Can you work these out from the model? Positions are in its coordinate system, mm. Coordinates: 2 decimals unless noted, no trailing zeros. Answer in a Markdown table with one row per item. Add a question column.
1. We'd pull the mould along X, two halves only. Please class faces 1 (the face through (0, -101.6, 35)), 2 (the face through (21.431, -36, 33)), 3 (the face through (0, -152.4, 47)), 4 (the face through (-1.24, -127.36, 44.37)): pulls with the +X half, pulls with the -X half, needs draft (parallel to the pull), parting line crosses it, or undercut.
2. Will these pins go through, and if not, where does the flat tip stop? pin 1 (9.5 mm diameter, centred on x = -3.5, z = 32.5, fed in from -Y); pin 2 (12 mm diameter, centred on x = -13.5, y = -12.5, fed in from +Z); pin 3 (2 mm diameter, centred on x = -5.5, z = 54.5, fed in from +Y).
3. If I drill on line 1 along Z through (x, y) = (0, -127); line 2 along Z through (x, y) = (0, -121.5); line 3 along Z through (x, y) = (-13.5, -98.5), over which ranges is the centre line in solid material (lowest first)? Write a range as [from, to].
from build123d import *

# Parameters (mm, degrees)
F1_DEPTH = 21.43125
F2_R     = 9.525
F3_DEPTH = 50.8
F8_DEPTH = 56.3


# Not quite as in the source:
# - ends of sketch curves that miss each other by under 0.0002 mm in the source are joined


with BuildPart() as f1:
    # F0 (on Right) → F1 (new body, symmetric)
    with BuildSketch(Plane.YZ):
        Polygon((-152.4, 69.85), (-152.4, 0), (152.4, 0), (152.4, 19.05), align=None)
    extrude(amount=F1_DEPTH, both=True)

    # F2 (on face) → F3 (cut)
    with BuildSketch(Plane.XZ.offset(152.4)):
        with Locations((0, 34.925)):
            Circle(F2_R)
    extrude(amount=-F3_DEPTH, mode=Mode.SUBTRACT)

    # F5 (on face) → F8 (cut)
    with BuildSketch(Plane.YZ.offset(21.43125)):
        with BuildLine():
            add(Edge.make_bspline(
                [(-94.6281477809, 51.2691959739), (-96.0952206694, 52.0179937663), (-97.562293558, 52.7667915588), (-99.0539994454, 53.491879309)],
                knots=[0, 0, 0, 0, 0.1035282224, 0.1035282224, 0.1035282224, 0.1035282224], degree=3))
            add(Edge.make_bspline(
                [(-94.6281477809, 51.2691959739), (-88.9739529123, 49.8775010567), (-83.3197580522, 48.4858061416), (-73.0600804397, 46.9911508307)],
                knots=[0, 0, 0, 0, 0.1804237123, 0.1804237123, 0.1804237123, 0.1804237123], degree=3))
            add(Edge.make_bspline(
                [(11.0397725003, 37.6377859426), (-20.7191231776, 41.240284312), (-53.8117553476, 44.4768553148), (-73.0600804397, 46.9911508307)],
                knots=[0.3821429542, 0.3821429542, 0.3821429542, 0.3821429542, 0.5639196837, 0.5639196837, 0.5639196837, 0.5639196837], degree=3))
            add(Edge.make_bspline(
                [(11.0397725003, 37.6377859426), (19.8326583687, 36.6506728683), (28.6537852654, 35.611343032), (37.2394360057, 34.5120057533)],
                knots=[0.5008053198, 0.5008053198, 0.5008053198, 0.5008053198, 0.5858071806, 0.5858071806, 0.5858071806, 0.5858071806], degree=3))
            add(Edge.make_bspline(
                [(151.5644788742, 15.5920218676), (140.3358248303, 17.736038831), (112.6697575345, 23.0186414795), (69.4706003693, 30.4232191611), (37.2394360057, 34.5120057533)],
                knots=[0, 0, 0, 0, 0.1343010577, 0.3309018237, 0.3309018237, 0.3309018237, 0.3309018237], degree=3))
            Line((151.5644788742, 15.5920218676), (-152.4, 15.5920218676))
            Line((-152.4, 15.5920218676), (-152.4, 0))
            Line((-152.4, 0), (152.4, 0))
            Line((152.4, 0), (152.4, 19.05))
            Line((152.4, 19.05), (-152.4, 69.85))
            Line((-152.4, 69.85), (-152.4, 58.510940522))
            add(Edge.make_bspline(
                [(-152.1597802639, 58.510940522), (-152.2398342689, 58.510940522), (-152.3198882739, 58.510940522), (-152.4, 58.510940522)],
                knots=[0, 0, 0, 0, 0.240162015, 0.240162015, 0.240162015, 0.240162015], degree=3))
            add(Edge.make_bspline(
                [(-126.880271242, 59.893312547), (-131.0252775202, 59.9641176604), (-141.283309107, 59.6280745769), (-148.0759439731, 58.9303957414), (-152.1597802639, 58.510940522)],
                knots=[0.8645812396, 0.8645812396, 0.8645812396, 0.8645812396, 0.9185841637, 1, 1, 1, 1], degree=3))
            add(Edge.make_bspline(
                [(-114.7441045161, 58.9132569857), (-118.4444301689, 59.5720764958), (-122.5362126789, 59.8541063708), (-126.880271242, 59.893312547)],
                knots=[0.431288265, 0.431288265, 0.431288265, 0.431288265, 0.6334912794, 0.6334912794, 0.6334912794, 0.6334912794], degree=3))
            add(Edge.make_bspline(
                [(-99.0539994454, 53.491879309), (-99.5844007901, 53.7839672826), (-103.1690308471, 55.7243154808), (-108.8461739052, 57.9235356565), (-114.7441045161, 58.9132569857)],
                knots=[0.7100922868, 0.7100922868, 0.7100922868, 0.7100922868, 0.7255634136, 0.8104095628, 0.8104095628, 0.8104095628, 0.8104095628], degree=3))
        make_face()
    extrude(amount=-F8_DEPTH, mode=Mode.SUBTRACT)


solid = f1.part
Answers follow:
| question | item | result |
|---|---|---|
| 1 | face 1 | undercut |
| 1 | face 2 | pulls with the +X half |
| 1 | face 3 | needs draft |
| 1 | face 4 | undercut |
| 2 | pin 1 | stops at y = -101.6 |
| 2 | pin 2 | stops at z = 40.88 |
| 2 | pin 3 | stops at y = -99.07 |
| 3 | line 1 | z = [15.59, 25.4], [44.45, 59.9] |
| 3 | line 2 | z = [15.59, 25.4], [44.45, 59.7] |
| 3 | line 3 | z = [15.59, 53.22] |
